Geometry: final body of the model. Coordinates: model frame, mm. A direction names the side the tool comes from. Coordinates: 2 decimals unless noted, no trailing zeros. Write each loop counter-clockwise with the first axis right and the second up, starting at its lowest first coordinate (ties: lowest second). Pieces come first, ordered by that corner, then holes. Notation, with made-up numbers: (11, -13.5) -> (21, -13.5) arc R26 ccw to (21, 10.5) -> close; hole circle Ø2 at (25, 78.5). An arc over 180 degrees is marked (long way). One line per item, written item: value.
Autodesk Inventor part; units mm, degrees
ref_plane "YZ Plane" through (0, 0, 0) normal (1, 0, 0) x (0, 1, 0)
ref_plane "XZ Plane" through (0, 0, 0) normal (0, 1, 0) x (-1, 0, 0)
ref_plane "XY Plane" through (0, 0, 0) normal (0, 0, 1) x (1, 0, 0)
sketch "Sketch1" plane through (0, 0, 0) normal (0, 0, 1) x (1, 0, 0)
  circle A0 centre (0, 0) radius 2.9845
  dimension "d0" = 5.969
extrude "Extrusion1" add sketch "Sketch1" along normal blind 12.7
sketch "Sketch2" plane through (0, 0, 12.7) normal (0, 0, 1) x (1, 0, 0)
  circle A0 centre (0, 0) radius 2.9845
  circle A1 centre (0, 0) radius 2.9845
  line L0 (1.4859, 2.5883) -> (1.4859, -2.5883)
  dimension "d3" = 1.4859
extrude "Extrusion2" cut sketch "Sketch2" against normal blind 10.0076 contours A0 L0 picked at (1.9854, 0)
sketch "Sketch3" plane through (0, 0, 0) normal (0, 0, -1) x (-1, 0, 0)
  circle A0 centre (0, 0) radius 2.9845
  circle A1 centre (0, 0) radius 1.4859
extrude "Extrusion3" add sketch "Sketch3" along normal blind 1.524 contours A1
chamfer "Chamfer1" distance 0.254 angle 45 1 edges at (-2.9845, 0, 12.7)
properties part number "shaft_encoder"
(1) Line query: line 1 (X direction, y = -1.2, z = 5.25); line 2 (Z direction, x = -1.75, y = -0.55); line 3 (Z direction, x = 1.95, y = 2). Output: solid intervals per line, ascending. Write a range as [from, to].
Responses:
line 1: x = [-2.73, 1.49]
line 2: z = [0, 12.7]
line 3: z = [0, 2.69]
(2) Reachability of faces 1 (the flat face through (0, 0, -1.524)), 2 (the flat face through (1.3, -1.3, 0)), 3 (the flat face through (2, 0, 2.692)) from +Z, -Z, +X, -X, +Y, -Y: full face, straight path, thin tool, end or side. Return the list, or none.
Responses:
face 1: -Z, +X, -X, +Y, -Y
face 2: -Z
face 3: +Z, +X, +Y, -Y
(3) Section D-D (z = 2.5). Return the cut outline in (x, y).
Responses:
outline: circle Ø5.97 at (0, 0)
(4) Section B-B (y = 0). Return the cut outline in (x, z).
Responses:
outline: (-2.98, 0) -> (-1.49, 0) -> (-1.49, -1.52) -> (1.49, -1.52) -> (1.49, 0) -> (2.98, 0) -> (2.98, 2.69) -> (1.49, 2.69) -> (1.49, 12.7) -> (-2.73, 12.7) -> (-2.98, 12.45) -> close
(5) Section A-A (x = 0). Return the cut outline in (y, z).
Responses:
outline: (-2.98, 0) -> (-1.49, 0) -> (-1.49, -1.52) -> (1.49, -1.52) -> (1.49, 0) -> (2.98, 0) -> (2.98, 12.45) -> (2.73, 12.7) -> (-2.73, 12.7) -> (-2.98, 12.45) -> close
(6) First-contact query: pin 1 (1.5 mm diameter, centred on x = -1, z = 10, fed in from -Y); pin 2 (3 mm diameter, centred on y = -1, z = 6.5, fed in from +X); pin 3 (1.6 mm diameter, centred on x = 2.5, y = -0.5, fed in from +Z). Flat tips, straight axial feed; report the tip coordinate or a pass-through.
Responses:
pin 1: stops at y = -2.97
pin 2: stops at x = 1.49
pin 3: stops at z = 2.69
(7) Section C-C (z = 11.25). Return the cut outline in (x, y).
Responses:
outline: (1.49, -2.59) -> (1.49, 2.59) arc R2.98 ccw (long way) to start
